```python
from build123d import *

# Parameters (mm, degrees)
BOSS_EXTRUDE1_DEPTH     = 124
FILLET1_R               = 6
SKETCH2_R               = 2.05
CUT_EXTRUDE1_DEPTH      = 125.643491607
LPATTERN1_COUNT         = 7
LPATTERN1_PITCH         = 8
MIRROR1_COPY_1_SKETCH_R = 2.05
MIRROR1_COPY_1_DEPTH    = 125.643491607
MIRROR1_COPY_2_SKETCH_R = 2.05
MIRROR1_COPY_2_DEPTH    = 125.643491607
MIRROR1_COPY_3_SKETCH_R = 2.05
MIRROR1_COPY_3_DEPTH    = 125.643491607
MIRROR1_COPY_4_SKETCH_R = 2.05
MIRROR1_COPY_4_DEPTH    = 125.643491607
MIRROR1_COPY_5_SKETCH_R = 2.05
MIRROR1_COPY_5_DEPTH    = 125.643491607


with BuildPart() as part:
    # Sketch1 → Boss-Extrude1 (new body)
    with BuildSketch(Plane.XY):
        Polygon((0, 0), (4, 0), (4, 2), (3, 2), (3, 10), (4, 10), (4, 12), (0, 12), align=None)
    extrude(amount=-BOSS_EXTRUDE1_DEPTH)

    # Fillet1
    fillet1_edges = [part.edges().sort_by_distance(p)[0] for p in [
        (2, 12, 0),
        (2, 0, 0),
        (2, 0, -124),
        (2, 12, -124),
    ]]
    fillet(fillet1_edges, radius=FILLET1_R - 0.0001)  # a hair under: the kernel refuses the full size

    # Sketch2 → Cut-Extrude1 (cut, through all)
    with BuildSketch(Plane.ZY):
        with Locations(Location((-118, 6, 0), (0, 0, 270))):
            Circle(SKETCH2_R)
    cut_extrude1 = extrude(amount=-CUT_EXTRUDE1_DEPTH, mode=Mode.SUBTRACT)

    # LPattern1: Cut-Extrude1 ×7, 1 skipped
    with Locations(*[(0, 0, i * LPATTERN1_PITCH) for i in range(1, LPATTERN1_COUNT) if i not in (5,)]):
        add(cut_extrude1, mode=Mode.SUBTRACT)

    # Mirror1: Cut-Extrude1 across plane
    add(cut_extrude1.mirror(Plane.XY.offset(-62)), mode=Mode.SUBTRACT)

    # Mirror1 copy 1 sketch → Mirror1 copy 1 (cut, through all)
    with BuildSketch(Plane(origin=(0, 0, -132), x_dir=(0, 0, -1), z_dir=(-1, 0, 0))):
        with Locations((-118, -6)):
            Circle(MIRROR1_COPY_1_SKETCH_R)
    extrude(amount=-MIRROR1_COPY_1_DEPTH, mode=Mode.SUBTRACT)

    # Mirror1 copy 2 sketch → Mirror1 copy 2 (cut, through all)
    with BuildSketch(Plane(origin=(0, 0, -140), x_dir=(0, 0, -1), z_dir=(-1, 0, 0))):
        with Locations((-118, -6)):
            Circle(MIRROR1_COPY_2_SKETCH_R)
    extrude(amount=-MIRROR1_COPY_2_DEPTH, mode=Mode.SUBTRACT)

    # Mirror1 copy 3 sketch → Mirror1 copy 3 (cut, through all)
    with BuildSketch(Plane(origin=(0, 0, -148), x_dir=(0, 0, -1), z_dir=(-1, 0, 0))):
        with Locations((-118, -6)):
            Circle(MIRROR1_COPY_3_SKETCH_R)
    extrude(amount=-MIRROR1_COPY_3_DEPTH, mode=Mode.SUBTRACT)

    # Mirror1 copy 4 sketch → Mirror1 copy 4 (cut, through all)
    with BuildSketch(Plane(origin=(0, 0, -156), x_dir=(0, 0, -1), z_dir=(-1, 0, 0))):
        with Locations((-118, -6)):
            Circle(MIRROR1_COPY_4_SKETCH_R)
    extrude(amount=-MIRROR1_COPY_4_DEPTH, mode=Mode.SUBTRACT)

    # Mirror1 copy 5 sketch → Mirror1 copy 5 (cut, through all)
    with BuildSketch(Plane(origin=(0, 0, -172), x_dir=(0, 0, -1), z_dir=(-1, 0, 0))):
        with Locations((-118, -6)):
            Circle(MIRROR1_COPY_5_SKETCH_R)
    extrude(amount=-MIRROR1_COPY_5_DEPTH, mode=Mode.SUBTRACT)


solid = part.part
```
Can you work these out from the model? Positions are in its coordinate system, mm. A direction names the side the tool comes from. Coordinates: 2 decimals unless noted, no trailing zeros. Order: outer loops, then holes, each group sorted by start corner. A loop starts at its lowest first (then second) coordinate and runs counter-clockwise, first axis right, second up. Notation, with made-up numbers: (59, 72.25) -> (114, 72.25) arc R21 cw to (114, 84.25) -> close; hole circle Ø2 at (-31, 54.25). An arc over 180 degrees is marked (long way). Write each question's results on one line, items separated by ' | '.
Item 1: I want a section at A-A, the plane z = -30. Write out the boundary of the cut face in (x, y).
Results are:
outline: (0, 0) -> (4, 0) -> (4, 2) -> (3, 2) -> (3, 3.95) -> (0, 3.95) -> close; (0, 8.05) -> (3, 8.05) -> (3, 10) -> (4, 10) -> (4, 12) -> (0, 12) -> close
Item 2: Which directions (+Z, -Z, +X, -X, +Y, -Y) give clear straight access to the entire face, cutting with the end or side of a thin tool? Please do faces 1 (the face through (1.479, 6.267, -115.967)), 2 (the face through (3, 6, -61)).
Results are:
face 1: +X, -X | face 2: +Z, -Z, +X
Item 3: If I drill on line 1 along Y through (x, z) = (3.8, -87); line 2 along Y through (x, z) = (2.2, -22); line 3 along X through (y, z) = (8.5, -82.5), over which ranges is the centre line in solid material (lowest first)?
Results are:
line 1: 0 to 2, 10 to 12 | line 2: 0 to 3.95, 8.05 to 12 | line 3: 0 to 3
Item 4: If we mould it in two halves opening along Y, with no side actions, what happens to faces 3 (the face through (1.479, 6.267, -107.967)), 4 (the face through (4, 1, -61)), 5 (the face through (1.48, 5.91, -51.95)), 6 (the face through (2.028, 1.711, -1.804))? For each: +Y half, -Y half, draft (parallel to the pull), parting line (faces both ways), or undercut.
Results are:
face 3: undercut | face 4: draft | face 5: undercut | face 6: -Y half
Item 5: I'm going to push flat-ended pins straight in: pin 1 Ø4 at (y, z) = (3, -81) entering from -X; pin 2 Ø4.5 at (y, z) = (6, -22) entering from +X; pin 3 Ø2 at (x, y) = (1.5, 9.5) entering from +Z. Where does each tip first touch, or does it pass through?
Results are:
pin 1: x = 0 | pin 2: x = 3 | pin 3: z = -0.55
Item 6: I want a section at B-B, the plane x = 2.1. Count the separate pieces of the cut face and the enclosed holes in it, then the cut area to 3 significant figures.
Results are:
separate pieces: 1 | enclosed holes: 12 | area: 1,300 mm²
